```python
from build123d import *

# Parameters (mm, degrees)
SKETCH1_W              = 501.65
SKETCH1_H              = 57.15
BOSS_EXTRUDE1_DEPTH    = 4.7625
BOSS_EXTRUDE2_DEPTH    = 4.7625
SKETCH23_W             = 100.33
SKETCH23_H             = 9.525
BOSS_EXTRUDE3_DEPTH    = 6.35
F_10_CLEARANCE_HOLE2_D = 5.1054
LPATTERN1_COUNT        = 6
LPATTERN1_PITCH        = 96.52
CUT_EXTRUDE6_REACH     = 275.327


with BuildPart() as part:
    # Sketch1 → Boss-Extrude1 (new, symmetric)
    with BuildSketch(Plane(origin=(0, 0, 0), x_dir=(1, 0, 0), z_dir=(0, 1, 0))):
        Rectangle(SKETCH1_W, SKETCH1_H)
    extrude(amount=BOSS_EXTRUDE1_DEPTH, both=True)

    # Sketch2 → Boss-Extrude2 (add, symmetric)
    with BuildSketch(Plane(origin=(0, 0, 0), x_dir=(1, 0, 0), z_dir=(0, 1, 0))):
        Polygon((161.925, -92.075), (161.925, -71.755), (250.825, -71.755), (250.825, -28.575), (-250.825, -28.575), (-250.825, -71.755), (-168.275, -71.755), (-168.275, -92.075), (-79.375, -92.075), (-79.375, -53.975), (60.325, -53.975), (60.325, -92.075), align=None)
    extrude(amount=BOSS_EXTRUDE2_DEPTH, both=True)

    # Sketch23 → Boss-Extrude3 (add)
    with BuildSketch(Plane.ZY.offset(250.825)):
        with Locations((21.59, 0)):
            Rectangle(SKETCH23_W, SKETCH23_H)
    boss_extrude3 = extrude(amount=BOSS_EXTRUDE3_DEPTH)

    # Mirror1: Boss-Extrude3 across plane
    add(boss_extrude3.mirror(Plane(origin=(0, 0, 0), x_dir=(0, 0, 1), z_dir=(1, 0, 0))))

    # #10 Clearance Hole2 (through all)
    with Locations(Plane(origin=(0, 4.7625, 0), x_dir=(1, 0, 0), z_dir=(0, 1, 0))):
        with Locations((241.3, 12.7)):
            f_10_clearance_hole2 = Hole(F_10_CLEARANCE_HOLE2_D / 2)

    # LPattern1: #10 Clearance Hole2 ×6
    with Locations(*[(-i * LPATTERN1_PITCH, 0, 0) for i in range(1, LPATTERN1_COUNT)]):
        add(f_10_clearance_hole2, mode=Mode.SUBTRACT)

    # Sketch40 → Cut-Extrude6 (cut, up to next)
    with BuildSketch(Plane(origin=(0, 4.7625, 0), x_dir=(1, 0, 0), z_dir=(0, 1, 0)), mode=Mode.PRIVATE) as cut_extrude6_sk1:
        with BuildLine():
            Line((-91.1479, -79.375), (-91.1479, -9.525))
            ThreePointArc((-91.1479, -9.525), (-88.9, -7.2771), (-86.6521, -9.525))
            Line((-86.6521, -9.525), (-86.6521, -79.375))
            ThreePointArc((-86.6521, -79.375), (-88.9, -81.6229), (-91.1479, -79.375))
        make_face()
    cut_extrude6_tool1 = extrude(cut_extrude6_sk1.sketch, amount=-CUT_EXTRUDE6_REACH, mode=Mode.PRIVATE) & part.part
    # Sketch40 → Cut-Extrude6 (cut, up to next)
    with BuildSketch(Plane(origin=(0, 4.7625, 0), x_dir=(1, 0, 0), z_dir=(0, 1, 0)), mode=Mode.PRIVATE) as cut_extrude6_sk2:
        with BuildLine():
            Line((67.6021, -79.375), (67.6021, -9.525))
            ThreePointArc((67.6021, -9.525), (69.85, -7.2771), (72.0979, -9.525))
            Line((72.0979, -9.525), (72.0979, -79.375))
            ThreePointArc((72.0979, -79.375), (69.85, -81.6229), (67.6021, -79.375))
        make_face()
    cut_extrude6_tool2 = extrude(cut_extrude6_sk2.sketch, amount=-CUT_EXTRUDE6_REACH, mode=Mode.PRIVATE) & part.part
    add(cut_extrude6_tool1.solids().sort_by_distance((-88.9, 4.7625, 44.45))[0], mode=Mode.SUBTRACT)
    add(cut_extrude6_tool2.solids().sort_by_distance((69.85, 4.7625, 44.45))[0], mode=Mode.SUBTRACT)


solid = part.part
```
Read the model definition and answer for the solid it produces. Units are mm, in the model's axes. A direction names the side the tool comes from. Coordinates: 2 decimals unless noted, no trailing zeros. Loops run counter-clockwise (first coordinate to the right, second up) from the corner with the lowest first, then second, coordinate; pieces in that order, holes last. Notation, with made-up numbers: (19, 28.5) -> (25, 28.5) arc R14 ccw to (25, 32.5) -> close; hole circle Ø11 at (28, 61). An arc over 180 degrees is marked (long way). Return JSON: item names as keys, results as strings.
Item 1: Find section D-D (x = 205.5). Determine the outline of the cut face in (y, z) (1 decimal).
Answers:
{"outline": "(-4.8, -28.6) -> (4.8, -28.6) -> (4.8, 71.8) -> (-4.8, 71.8) -> close"}
Item 2: Find the intervals of material crossed by probe 1 along X at (y, z) = (-4.5, 10.5) (3 decimals); probe 2 along X at (y, z) = (-4, 58) (3 decimals); probe 3 along Z at (x, y) = (241.3, -2) (3 decimals), in increasing order.
Answers:
{"probe 1": "x = -257.175 to -91.148, -86.652 to 67.602, 72.098 to 257.175", "probe 2": "x = -257.175 to -91.148, -86.652 to -79.375, 60.325 to 67.602, 72.098 to 257.175", "probe 3": "z = -28.575 to -15.253, -10.147 to 71.755"}
Item 3: Find section B-B (y = 0). Count the separate pieces of the cut face and the enclosed holes in it, plus the area to 3 significant figures.
Answers:
{"separate pieces": "1", "enclosed holes": "8", "area": "52,200 mm2"}
Item 4: For a pull along Z with two mould halves and no side action, classify faces 5 (the flat face through (67.602, 0, 45)), 6 (the flat face through (-257.175, 0, 21)), 7 (the flat face through (110, 0, 92.075)) as +Z half, -Z half, draft (parallel to the pull), parting line (faces both ways), or undercut.
Answers:
{"face 5": "undercut", "face 6": "draft", "face 7": "+Z half"}
Item 5: Find section C-C (x = -39). Determine the outline of the cut face in (y, z) (1 decimal).
Answers:
{"outline": "(-4.8, -28.6) -> (4.8, -28.6) -> (4.8, 54) -> (-4.8, 54) -> close"}
Item 6: For faces 1 (the flat face through (-91.148, 0, 45)), 2 (the flat face through (-168.275, 0, 82)), 3 (the flat face through (161.925, 0, 82)), 4 (the flat face through (-79.375, 0, 73)), determine the directions among +Z, -Z, +X, -X, +Y, -Y from which every point of the face is accessible in a straight line to the end or side of a thin tool.
Answers:
{"face 1": "+Y, -Y", "face 2": "+Z, -X, +Y, -Y", "face 3": "+Z, +X, +Y, -Y", "face 4": "+Z, +Y, -Y"}
Item 7: Find section A-A (z = 19). Determine the outline of the cut face in (x, y) (1 decimal), plus the area to 3 significant figures.
Answers:
{"outline": "(-257.2, -4.8) -> (-91.1, -4.8) -> (-91.1, 4.8) -> (-257.2, 4.8) -> close; (-86.7, -4.8) -> (67.6, -4.8) -> (67.6, 4.8) -> (-86.7, 4.8) -> close; (72.1, -4.8) -> (257.2, -4.8) -> (257.2, 4.8) -> (72.1, 4.8) -> close", "area": "4,810 mm2"}
Item 8: Flat-ended cylindrical pins translate along their axes: P1, Ø3, axis at x = -226, y = 0, coming from the +Z side (3 decimals); P2, Ø3, axis at x = -64.5, y = 2.5, coming from the +Z side (3 decimals); P3, Ø6.5, axis at x = 241.3, z = -12.7, coming from the +Y side; P4, Ø3, axis at x = 48.26, z = -12.7, coming from the +Y side. Find the tip coordinate at first contact, or state that the pin passes through.
Answers:
{"P1": "stops at z = 71.755", "P2": "stops at z = 53.975", "P3": "stops at y = 4.76", "P4": "passes through"}
